Verification items for the finished model (mm, model axes). A direction names the side the tool comes from. Coordinates: 2 decimals unless noted, no trailing zeros. Loops run counter-clockwise (first coordinate to the right, second up) from the corner with the lowest first, then second, coordinate; pieces in that order, holes last. Notation, with made-up numbers: (0, 76) -> (7, 76) arc R5 ccw to (7, 83) -> close; hole circle Ø5 at (-17, 19). An arc over 180 degrees is marked (long way). Write item = value, one per line.
```python
from build123d import *

# Parameters (mm, degrees)
F0_W     = 47
F0_H     = 40
F0_R     = 7
F1_DEPTH = 16
F2_W     = 3.5
F2_H     = 13
F3_DEPTH = 40.001
F4_R     = 13
F4_R_2   = 7
F5_DEPTH = 12.5
F6_R     = 16
F6_R_2   = 13
F7_DEPTH = 12


with BuildPart() as f1:
    # F0 (on Front) → F1 (new body)
    with BuildSketch(Plane.XZ):
        Rectangle(F0_W, F0_H)
        Circle(F0_R, mode=Mode.SUBTRACT)
    extrude(amount=F1_DEPTH)

    # F2 (on face) → F3 (cut, through all)
    with BuildSketch(Plane.XY.offset(20)):
        with Locations((-21.75, -6.5)):
            Rectangle(F2_W, F2_H)
        with Locations((21.75, -6.5)):
            Rectangle(F2_W, F2_H)
    extrude(amount=-F3_DEPTH, mode=Mode.SUBTRACT)

    # F4 (on face) → F5 (cut)
    with BuildSketch(Plane.XZ.offset(16)):
        Circle(F4_R)
        Circle(F4_R_2, mode=Mode.SUBTRACT)
    extrude(amount=-F5_DEPTH, mode=Mode.SUBTRACT)

    # F6 (on face) → F7 (cut)
    with BuildSketch(Plane.XZ.offset(16)):
        Circle(F6_R)
        Circle(F6_R_2, mode=Mode.SUBTRACT)
    extrude(amount=-F7_DEPTH, mode=Mode.SUBTRACT)


solid = f1.part
```
1) Sectioned sample at D-D, the plane z = 6. Record the cut outline in (x, y).
Ans:
outline = (-23.5, -16) -> (-14.83, -16) -> (-14.83, -4) -> (-11.53, -4) -> (-11.53, -3.5) -> (-3.61, -3.5) -> (-3.61, 0) -> (-20, 0) -> (-20, -13) -> (-23.5, -13) -> close; (3.61, -3.5) -> (11.53, -3.5) -> (11.53, -4) -> (14.83, -4) -> (14.83, -16) -> (23.5, -16) -> (23.5, -13) -> (20, -13) -> (20, 0) -> (3.61, 0) -> close
2) Tool access check on faces 4 (the face through (-20, -7, 0)), 5 (the face through (22, -13, 0)), 6 (the face through (-1.3, -4, 13.1)). Record the directions out of +Z, -Z, +X, -X, +Y, -Y that give a thin tool (end or side, any length) a straight path to the whole face; none if there is none.
Ans:
face_4 = +Z, -Z, -X, +Y
face_5 = +Z, -Z, +X, +Y
face_6 = -Y
3) Depth check by flat-ended pin: pin 1 Ø18 at (x, z) = (0, 0) entering from -Y; pin 2 Ø1.5 at (y, z) = (-10.5, 15) entering from +X; pin 3 Ø3 at (x, z) = (22.5, -7.5) entering from +Y. Enter the tip coordinate at first touch or a pass-through.
Ans:
pin_1 = -3.5
pin_2 = 20
pin_3 = -13
4) Sectioned sample at C-C, the plane y = -9.5. Record the cut outline in (x, z), plus the area to 3 significant figures.
Ans:
outline = (-20, -20) -> (20, -20) -> (20, 20) -> (-20, 20) -> close; hole circle Ø32 at (0, 0)
area = 796 mm2
5) Release check for a two-part mould opening along X. For faces 1 (the face through (20, -7, 0)), 2 (the face through (-22, -13, 0)), 3 (the face through (-10.316, -3.754, -7.91)) record: pulls with the +X half, pulls with the -X half, needs draft (parallel to the pull), parting line crosses it, or undercut.
Ans:
face_1 = pulls with the +X half
face_2 = needs draft
face_3 = undercut
6) Sectioned sample at A-A, the plane x = 0. Record the cut outline in (y, z), plus the area to 3 significant figures.
Ans:
outline = (-16, -20) -> (0, -20) -> (0, -7) -> (-3.5, -7) -> (-3.5, -13) -> (-4, -13) -> (-4, -16) -> (-16, -16) -> close; (-16, 16) -> (-4, 16) -> (-4, 13) -> (-3.5, 13) -> (-3.5, 7) -> (0, 7) -> (0, 20) -> (-16, 20) -> close
area = 194 mm2
7) Sectioned sample at B-B, the plane z = 0. Record the cut outline in (x, y).
Ans:
outline = (-23.5, -16) -> (-16, -16) -> (-16, -4) -> (-13, -4) -> (-13, -3.5) -> (-7, -3.5) -> (-7, 0) -> (-20, 0) -> (-20, -13) -> (-23.5, -13) -> close; (7, -3.5) -> (13, -3.5) -> (13, -4) -> (16, -4) -> (16, -16) -> (23.5, -16) -> (23.5, -13) -> (20, -13) -> (20, 0) -> (7, 0) -> close
8) Material ranges on line 1 (Z direction, x = 0, y = -1.3); line 2 (Z direction, x = 0, y = -3.85); line 3 (Y direction, x = -2, z = -14.5), recorded low to high.
Ans:
line_1 = -20 to -7, 7 to 20
line_2 = -20 to -13, 13 to 20
line_3 = -4 to 0
